Input: part model. Units: mm. Frame: model coordinates. A direction names the side the tool comes from. Give positions to 0.01 mm unless a question says otherwise; leave off trailing zeros. Loops run counter-clockwise (first coordinate to the right, second up) from the corner with the lowest first, then second, coordinate; pieces in that order, holes last. Notation, with made-up numbers: (12, 44.25) -> (58, 44.25) arc R21 cw to (58, 52.25) -> close; hole circle Ø1 at (-6.75, 67.25). An arc over 180 degrees is marked (long way). Answer as a JSON object with one key per item and string values. Group by question number.
```python
from build123d import *

# Parameters (mm, degrees)
SKETCH1_R              = 12.7
SKETCH1_R_2            = 8.73125
BOSS_EXTRUDE1_DEPTH    = 4.7625
BOSS_EXTRUDE5_DEPTH    = 4.7625
BOSS_EXTRUDE2_DEPTH    = 4.7625
BOSS_EXTRUDE2_2_DEPTH  = 4.7625
BOSS_EXTRUDE3_DEPTH    = 12.7
FILLET2_R              = 25.4
F_10_CLEARANCE_HOLE1_D = 5.1054
CONVERT_SOLID1_START   = -12.7
CONVERT_SOLID1_DEPTH   = 25.4
CONVERT_SOLID1_2_DEPTH = 25.4
CONVERT_SOLID1_3_DEPTH = 25.4
CONVERT_SOLID1_4_DEPTH = 25.4


# Read off the part's stored shape, not the designer's step: Convert-Solid1
with BuildPart() as part:
    # Sketch1 → Boss-Extrude1 (new body)
    with BuildSketch(Plane(origin=(0, 0, 0), x_dir=(1, 0, 0), z_dir=(0, 1, 0))):
        with Locations(Location((0, 0, 0), (0, 0, 90))):
            Circle(SKETCH1_R)
        with Locations(Location((0, 0, 0), (0, 0, 90))):
            Circle(SKETCH1_R_2, mode=Mode.SUBTRACT)
    extrude(amount=BOSS_EXTRUDE1_DEPTH)

    # Sketch1<5> → Boss-Extrude5 (add)
    with BuildSketch(Plane(origin=(0, 0, 0), x_dir=(1, 0, 0), z_dir=(0, 1, 0))):
        with BuildLine():
            Line((-25.256245596, 4.166855334), (-16.412307744, -19.643746575))
            Line((-16.412307744, -19.643746575), (0, -13.547746556))
            Line((0, -13.547746556), (-4.421968926, -11.905300955))
            ThreePointArc((-4.421968926, -11.905300955), (-12.7, 0), (-4.421968926, 11.905300955))
            Line((-4.421968926, 11.905300955), (-25.256245596, 4.166855334))
        make_face()
        with BuildLine():
            Line((-4.421968926, -11.905300955), (0, -13.547746556))
            Line((0, -13.547746556), (4.421968926, -11.905300955))
            ThreePointArc((4.421968926, -11.905300955), (0, -12.7), (-4.421968926, -11.905300955))
        make_face()
        with BuildLine():
            Line((4.421968926, -11.905300955), (0, -13.547746556))
            Line((0, -13.547746556), (16.412307744, -19.643746575))
            Line((16.412307744, -19.643746575), (25.256245596, 4.166855334))
            Line((25.256245596, 4.166855334), (4.421968926, 11.905300955))
            ThreePointArc((4.421968926, 11.905300955), (10.427104233, 7.250206709), (12.7, 0))
            ThreePointArc((12.7, 0), (10.427104233, -7.250206709), (4.421968926, -11.905300955))
        make_face()
    extrude(amount=BOSS_EXTRUDE5_DEPTH)



with BuildPart() as body_2:
    # Sketch3 → Boss-Extrude2 (new body)
    with BuildSketch(Plane(origin=(0, -35.179, 0), x_dir=(1, 0, 0), z_dir=(0, 1, 0))):
        with BuildLine():
            Line((-106.61799321, -26.053222351), (-115.546968926, -29.369699045))
            ThreePointArc((-115.546968926, -29.369699045), (-123.030300955, -45.696968926), (-106.703031074, -53.180300955))
            Line((-106.703031074, -53.180300955), (-97.774055358, -49.86382426))
            Line((-97.774055358, -49.86382426), (-106.61799321, -26.053222351))
        make_face()
    extrude(amount=BOSS_EXTRUDE2_DEPTH)


with BuildPart() as body_3:
    # Sketch3 → Boss-Extrude2 2 (new body)
    with BuildSketch(Plane(origin=(0, -35.179, 0), x_dir=(1, 0, 0), z_dir=(0, 1, 0))):
        with BuildLine():
            ThreePointArc((115.546968926, -29.369699045), (123.030300955, -45.696968926), (106.703031074, -53.180300955))
            Line((106.703031074, -53.180300955), (97.774055358, -49.86382426))
            Line((97.774055358, -49.86382426), (106.61799321, -26.053222351))
            Line((106.61799321, -26.053222351), (115.546968926, -29.369699045))
        make_face()
    extrude(amount=BOSS_EXTRUDE2_2_DEPTH)


with BuildPart() as part_1:
    add(part.part)

    add(body_2.part)  # Boss-Extrude3 merges body 2
    # Sketch4 → Boss-Extrude3 (add, symmetric)
    with BuildSketch(Plane(origin=(0, 0, 0), x_dir=(0.9374252720097653, 0, -0.34818652960362706), z_dir=(0.34818652960362706, 0, 0.9374252720097653))):
        Polygon((-109.937239497, -30.4165), (-109.017782361, -30.4165), (-109.017782361, -35.179), (-21.305542864, 0), (-22.225, 0), (-22.225, 4.7625), align=None)
    boss_extrude3 = extrude(amount=BOSS_EXTRUDE3_DEPTH, both=True)

    # Mirror1: Boss-Extrude3 across plane
    add(boss_extrude3.mirror(Plane(origin=(0, 0, 0), x_dir=(0, 0, 1), z_dir=(1, 0, 0))))


with BuildPart() as body_3_1:
    add(body_3.part)

    # Combine1: union part
    add(part_1.part)

    # Fillet2
    fillet2_edges = [body_3_1.edges().sort_by_distance(p)[0] for p in [
        (0, 2.38125, 13.547746556),
    ]]
    fillet(fillet2_edges, radius=FILLET2_R)

    # #10 Clearance Hole1 (through all)
    with Locations(Plane(origin=(0, -30.4165, 0), x_dir=(1, 0, 0), z_dir=(0, 1, 0))):
        with Locations((-111.125, -41.275), (111.125, -41.275)):
            Hole(F_10_CLEARANCE_HOLE1_D / 2)

    # Convert-Solid1 outline → Convert-Solid1 (add)
    with BuildSketch(Plane(origin=(0, 0, 0), x_dir=(0.9374252720097653, 0, -0.3481865296036272), z_dir=(0.34818652960362717, 0, 0.9374252720097654)).offset(CONVERT_SOLID1_START)):
        with BuildLine():
            ThreePointArc((-109.083861056, -30.074233056), (-109.953910301, -30.330150456), (-110.856696633, -30.4165))
            Line((-110.856696633, -30.4165), (-109.937239497, -30.4165))
            Line((-109.937239497, -30.4165), (-109.083861056, -30.074233056))
        make_face()
        with BuildLine():
            Line((-21.305542864, 0), (-22.158921305, -0.342266944))
            ThreePointArc((-22.158921305, -0.342266944), (-21.28887206, -0.086349544), (-20.386085729, 0))
            Line((-20.386085729, 0), (-21.305542864, 0))
        make_face()
    extrude(amount=CONVERT_SOLID1_DEPTH)

    # Convert-Solid1 2 outline → Convert-Solid1 2 (add)
    with BuildSketch(Plane(origin=(0, 0, 0), x_dir=(0.9374252720097653, 0, 0.3481865296036272), z_dir=(0.34818652960362717, 0, -0.9374252720097654)).offset(CONVERT_SOLID1_START)):
        with BuildLine():
            ThreePointArc((109.083861056, 30.074233056), (109.953910301, 30.330150456), (110.856696633, 30.4165))
            Line((110.856696633, 30.4165), (109.937239497, 30.4165))
            Line((109.937239497, 30.4165), (109.083861056, 30.074233056))
        make_face()
        with BuildLine():
            Line((21.305542864, 0), (22.158921305, 0.342266944))
            ThreePointArc((22.158921305, 0.342266944), (21.28887206, 0.086349544), (20.386085729, 0))
            Line((20.386085729, 0), (21.305542864, 0))
        make_face()
    extrude(amount=CONVERT_SOLID1_2_DEPTH)

    # Convert-Solid1 3 outline → Convert-Solid1 3 (cut)
    with BuildSketch(Plane(origin=(0, 0, 0), x_dir=(0.9374252720097653, 0, -0.3481865296036272), z_dir=(0.34818652960362717, 0, 0.9374252720097654)).offset(CONVERT_SOLID1_START)):
        with BuildLine():
            Line((-22.225, 4.7625), (-23.931756882, 4.077966112))
            ThreePointArc((-23.931756882, 4.077966112), (-22.191658392, 4.589800912), (-20.386085729, 4.7625))
            Line((-20.386085729, 4.7625), (-22.225, 4.7625))
        make_face()
        with BuildLine():
            ThreePointArc((-107.31102548, -34.494466112), (-109.05112397, -35.006300912), (-110.856696633, -35.179))
            Line((-110.856696633, -35.179), (-109.017782361, -35.179))
            Line((-109.017782361, -35.179), (-107.31102548, -34.494466112))
        make_face()
    extrude(amount=CONVERT_SOLID1_3_DEPTH, mode=Mode.SUBTRACT)

    # Convert-Solid1 4 outline → Convert-Solid1 4 (cut)
    with BuildSketch(Plane(origin=(0, 0, 0), x_dir=(0.9374252720097653, 0, 0.3481865296036272), z_dir=(0.34818652960362717, 0, -0.9374252720097654)).offset(CONVERT_SOLID1_START)):
        with BuildLine():
            Line((22.225, -4.7625), (23.931756882, -4.077966112))
            ThreePointArc((23.931756882, -4.077966112), (22.191658392, -4.589800912), (20.386085729, -4.7625))
            Line((20.386085729, -4.7625), (22.225, -4.7625))
        make_face()
        with BuildLine():
            ThreePointArc((107.31102548, 34.494466112), (109.05112397, 35.006300912), (110.856696633, 35.179))
            Line((110.856696633, 35.179), (109.017782361, 35.179))
            Line((109.017782361, 35.179), (107.31102548, 34.494466112))
        make_face()
    extrude(amount=CONVERT_SOLID1_4_DEPTH, mode=Mode.SUBTRACT)


solid = body_3_1.part
```
Q1. Section C-C on x = 56. Return the cut outline in (y, z).
Q2. Section A-A on x = 0. Return the cut outline in (y, z).
Q3. Ray query, probe 1 along Y at (x, z) = (-4.5, 15); probe 2 along Y at (x, z) = (106.5, 33). Return the intervals inside material, ascending.
Q4. Pin query (flat end, axial travel): pin 1 Ø10 at (x, z) = (65.5, 15.5) entering from -Y; pin 2 Ø6 at (x, z) = (-62.5, 34.5) entering from +Y; pin 3 Ø16 at (x, z) = (7, 10.5) entering from -Y. Return the tip coordinate at first contact, or that it passes through.
Q5. Set-up query: faces 1 (the face through (19.91, -0.09, 7.58)), 2 (the face through (0.126, 2.415, 15.244)). Return all of +Z, -Z, +X, -X, +Y, -Y with unobstructed straight access to the full face (end or side cutting, diameter ignored); none if empty.
Q6. Pull-direction query (X, two-part tool) for faces 3 (the face through (-115, -30.417, 43)), 4 (the face through (-61.73, -12.76, 23.12)), 5 (the face through (61.181, -17.657, 22.914)); classes: +X half, -X half, draft (parallel to the pull), parting line (faces both ways), or undercut.
Q7. Section B-B on y = -6. Return the cut outline in (x, z), then the cut area to 3 significant figures.
Numbers:
{
 "1": {"outline": "(-17.31, 34.35) -> (-13.52, 7.25) -> (-8.39, 7.25) -> (-12.17, 34.35) -> close"},
 "2": {"outline": "(0, -12.7) -> (4.76, -12.7) -> (4.76, -8.73) -> (0, -8.73) -> close; (0, 8.73) -> (4.76, 8.73) -> (4.76, 15.24) -> (0, 15.24) -> close"},
 "3": {"probe 1": "y = 0 to 4.76", "probe 2": "y = -35.18 to -30.42"},
 "4": {"pin 1": "stops at y = -20.25", "pin 2": "stops at y = -13.44", "pin 3": "stops at y = 0"},
 "5": {"face 1": "-Z, -Y", "face 2": "+Z, +Y, -Y"},
 "6": {"face 3": "draft", "face 4": "-X half", "face 5": "undercut"},
 "7": {"outline": "(-50.41, 5.18) -> (-38.42, 0.72) -> (-29.57, 24.53) -> (-41.57, 28.99) -> close; (29.57, 24.53) -> (38.42, 0.72) -> (50.41, 5.18) -> (41.57, 28.99) -> close", "area": "650 mm²"}
}
